Build history of the part. All positions in model axes, mm. A direction names the side the tool comes from. Give positions to 0.01 mm unless a question says otherwise; leave off trailing zeros. Order: outer loops, then holes, each group sorted by start corner. A loop starts at its lowest first (then second) coordinate and runs counter-clockwise, first axis right, second up. Notation, with made-up numbers: (-28.5, -38) - (-17.5, -38) arc R15 ccw to (-17.5, -30) - close; hole circle Ø6 at (-25, 53.25). An arc over 180 degrees is marked (long way). Answer in a Markdown table with one row per item.
```python
from build123d import *

# Parameters (mm, degrees)
F0_R     = 48.166826
F1_DEPTH = 1.750732
F3_R     = 4.01791
F3_R_2   = 4.772257
F3_R_3   = 4.448486
F3_R_4   = 3.51804
F4_DEPTH = 134.586155


with BuildPart() as f1:
    # F0 (on Top) → F1 (new body)
    with BuildSketch(Plane.XY):
        Circle(F0_R)
    extrude(amount=F1_DEPTH)

    # F3 (on face) → F4 (join)
    with BuildSketch(Plane(origin=(0, 0, 0), x_dir=(1, 0, 0), z_dir=(0, 0, -1))):
        with Locations((-20.741474, -22.985213)):
            Circle(F3_R)
        with Locations((-28.151382, 21.579884)):
            Circle(F3_R_2)
        with Locations((22.852417, 22.529926)):
            Circle(F3_R_3)
        with Locations((23.104079, -28.06554)):
            Circle(F3_R_4)
    extrude(amount=F4_DEPTH)


solid = f1.part
```
1. Cut at C-C on z = -6.5. Write the cut outline in (x, y), and give its area (3 significant figures).
Check result:
| item | result |
|---|---|
| outline | circle Ø9.54 at (-28.15, -21.58); circle Ø8.04 at (-20.74, 22.99); circle Ø8.9 at (22.85, -22.53); circle Ø7.04 at (23.1, 28.07) |
| area | 223 mm² |
2. Which spindle directions (+Z, -Z, +X, -X, +Y, -Y) get a long thin tool onto all of the face, cutting with end or side? Do faces 4 (the face through (-1, 1, 1.751)), 5 (the face through (22.27, -26.94, -66.35)). Say none if no direction does.
Check result:
| item | result |
|---|---|
| face 4 | +Z, +X, -X, +Y, -Y |
| face 5 | -Z |
3. Cut at A-A on x = -28.5. Write the cut outline in (y, z).
Check result:
| item | result |
|---|---|
| outline | (-38.83, 0) - (-26.34, 0) - (-26.34, -134.59) - (-16.82, -134.59) - (-16.82, 0) - (38.83, 0) - (38.83, 1.75) - (-38.83, 1.75) - close |
4. Cut at B-B on y = 0. Write the cut outline in (x, z), and give its area (3 significant figures).
Check result:
| item | result |
|---|---|
| outline | (-48.17, 0) - (48.17, 0) - (48.17, 1.75) - (-48.17, 1.75) - close |
| area | 169 mm² |
5. Probe line 1 (Z direction, x = 11, y = 26); line 2 (X direction, y = 23, z = -65); line 3 (X direction, y = -21, z = -71.5). List the from-to ranges inside material, lowest first.
Check result:
| item | result |
|---|---|
| line 1 | z = 0 to 1.75 |
| line 2 | x = -24.76 to -16.72 |
| line 3 | x = -32.89 to -23.41, 18.68 to 27.03 |
6. Two-plate mould, pull along X, no slides. Class faces 1 (the face through (-28, -22, -134.586)), 2 (the face through (-31.94, -18.68, -66.35)), 3 (the face through (-10.44, -47.02, 0.86)): +X half, -X half, draft (parallel to the pull), parting line (faces both ways), or undercut.
Check result:
| item | result |
|---|---|
| face 1 | draft |
| face 2 | undercut |
| face 3 | parting line |
7. Drop flat-ended pins along their axis: P1, Ø6, axis at x = -31.5, z = -91.5, coming from the -Y side; P2, Ø4, axis at x = 31, y = -22, coming from the -Z side; P3, Ø10, axis at y = -14.5, z = -23, coming from the -X side. Give the stop position or say it passes through.
Check result:
| item | result |
|---|---|
| P1 | stops at y = -26.34 |
| P2 | stops at z = 0 |
| P3 | stops at x = -32.45 |
8. Cut at D-D on y = -24.5. Write the cut outline in (x, z).
Check result:
| item | result |
|---|---|
| outline | (-41.47, 0) - (-31.93, 0) - (-31.93, -134.59) - (-24.38, -134.59) - (-24.38, 0) - (18.86, 0) - (18.86, -134.59) - (26.84, -134.59) - (26.84, 0) - (41.47, 0) - (41.47, 1.75) - (-41.47, 1.75) - close |
